Can you work these out from the model? Positions are in its coordinate system, mm. Coordinates: 2 decimals unless noted, no trailing zeros. Write each loop counter-clockwise with the first axis right and the second up, starting at its lowest first coordinate (ties: lowest second). Pieces come first, ordered by that corner, then holes. Notation, with made-up numbers: (-21.5, 79.25) -> (11.5, 79.25) arc R20 cw to (11.5, 88.25) -> close; hole circle Ø11 at (-33, -30). An arc over 180 degrees is marked (long way). Use one line per item in the form item = value.
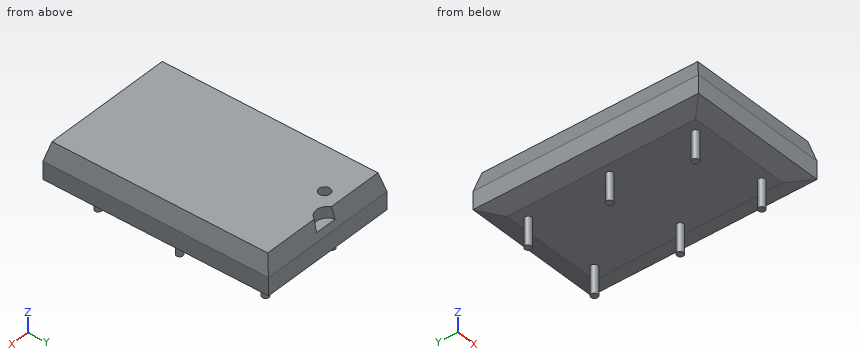
```python
from build123d import *
from OCP.BRepFilletAPI import BRepFilletAPI_MakeChamfer

# Parameters (mm, degrees)
SKETCH_2_W          = 12.6
SKETCH_2_H          = 20.2
EXTRUDE_1_DEPTH     = 3.68
CHAMFER_1_SIZE      = 1.65
CHAMFER_1_SIZE2     = 0.442116168
SKETCH_6_R          = 1
SKETCH_6_R_2        = 0.5
CUT_EXTRUDE_1_DEPTH = 1
SKETCH_7_R          = 0.3
EXTRUDE_2_DEPTH     = 2.5


with BuildPart() as part:
    # Эскиз2 → Вытянуть1 (new body)
    with BuildSketch(Plane.XY.offset(4.32)):
        with Locations((4.13, -7.62)):
            Rectangle(SKETCH_2_W, SKETCH_2_H)
    extrude(amount=-EXTRUDE_1_DEPTH)

    # Фаска1: one chamfer whose edges measure the first distance from different faces: ONE call of the kernel's chamfer builder (chamfer() names one face for all edges)
    chamfer_1_edges_1 = [part.edges().sort_by_distance(p)[0] for p in [
        (10.43, -7.62, 0.64),
        (4.13, 2.48, 0.64),
        (-2.17, -7.62, 0.64),
        (4.13, -17.72, 0.64),
    ]]
    chamfer_1_side_1 = [part.faces().sort_by_distance(p)[0] for p in [
        (4.13, -7.62, 0.64),
    ]]
    chamfer_1_edges_2 = [part.edges().sort_by_distance(p)[0] for p in [
        (4.13, 2.48, 4.32),
    ]]
    chamfer_1_side_2 = [part.faces().sort_by_distance(p)[0] for p in [
        (4.13, 2.48, 2.48),
    ]]
    chamfer_1_edges_3 = [part.edges().sort_by_distance(p)[0] for p in [
        (10.43, -7.62, 4.32),
    ]]
    chamfer_1_side_3 = [part.faces().sort_by_distance(p)[0] for p in [
        (10.43, -7.62, 2.48),
    ]]
    chamfer_1_edges_4 = [part.edges().sort_by_distance(p)[0] for p in [
        (4.13, -17.72, 4.32),
    ]]
    chamfer_1_side_4 = [part.faces().sort_by_distance(p)[0] for p in [
        (4.13, -17.72, 2.48),
    ]]
    chamfer_1_edges_5 = [part.edges().sort_by_distance(p)[0] for p in [
        (-2.17, -7.62, 4.32),
    ]]
    chamfer_1_side_5 = [part.faces().sort_by_distance(p)[0] for p in [
        (-2.17, -7.62, 2.48),
    ]]
    chamfer_1 = BRepFilletAPI_MakeChamfer(part.part.solid().wrapped)
    for e in chamfer_1_edges_1:
        chamfer_1.Add(CHAMFER_1_SIZE, CHAMFER_1_SIZE2, e.wrapped, chamfer_1_side_1[0].wrapped)  # the first distance lies on this face
    for e in chamfer_1_edges_2:
        chamfer_1.Add(CHAMFER_1_SIZE, CHAMFER_1_SIZE2, e.wrapped, chamfer_1_side_2[0].wrapped)  # the first distance lies on this face
    for e in chamfer_1_edges_3:
        chamfer_1.Add(CHAMFER_1_SIZE, CHAMFER_1_SIZE2, e.wrapped, chamfer_1_side_3[0].wrapped)  # the first distance lies on this face
    for e in chamfer_1_edges_4:
        chamfer_1.Add(CHAMFER_1_SIZE, CHAMFER_1_SIZE2, e.wrapped, chamfer_1_side_4[0].wrapped)  # the first distance lies on this face
    for e in chamfer_1_edges_5:
        chamfer_1.Add(CHAMFER_1_SIZE, CHAMFER_1_SIZE2, e.wrapped, chamfer_1_side_5[0].wrapped)  # the first distance lies on this face
    add(Compound.cast(chamfer_1.Shape()), mode=Mode.REPLACE)

    # Эскиз6 → Вырез-Вытянуть1 (cut)
    with BuildSketch(Plane.XY.offset(4.32)):
        with Locations((4.13, 2.48)):
            Circle(SKETCH_6_R)
        with Locations((2.197434959, 0.574075773)):
            Circle(SKETCH_6_R_2)
    extrude(amount=-CUT_EXTRUDE_1_DEPTH, mode=Mode.SUBTRACT)

    # Эскиз7 → Вытянуть2 (add)
    with BuildSketch(Plane(origin=(0, 0, 0.64), x_dir=(-1, 0, 0), z_dir=(0, 0, -1))):
        with Locations(Location((-7.88, -7.62, 0), (0, 0, 180))):
            Circle(SKETCH_7_R)
        with Locations(Location((-7.653482529, -0.12, 0), (0, 0, 180))):
            Circle(SKETCH_7_R)
        with Locations(Location((-7.653482529, -15.12, 0), (0, 0, 180))):
            Circle(SKETCH_7_R)
        with Locations(Location((-0.606517471, -15.12, 0), (0, 0, 180))):
            Circle(SKETCH_7_R)
        with Locations(Location((-0.606517471, -0.12, 0), (0, 0, 180))):
            Circle(SKETCH_7_R)
        with Locations(Location((-0.38, -7.62, 0), (0, 0, 180))):
            Circle(SKETCH_7_R)
    extrude(amount=EXTRUDE_2_DEPTH)


solid = part.part
```
Q1. Suppose I cut it at D-D (x = -1). Write out the boundary of the cut face in (y, z).
Return value:
outline = (-17.72, 1.08) -> (-16.55, 0.77) -> (1.31, 0.77) -> (2.48, 1.08) -> (2.48, 2.67) -> (2.04, 4.32) -> (-17.28, 4.32) -> (-17.72, 2.67) -> close
Q2. Suppose I cut it at B-B (y = -15.12). Write out the boundary of the cut face in (x, z).
Return value:
outline = (-2.17, 1.08) -> (-0.52, 0.64) -> (0.31, 0.64) -> (0.31, -1.86) -> (0.91, -1.86) -> (0.91, 0.64) -> (7.35, 0.64) -> (7.35, -1.86) -> (7.95, -1.86) -> (7.95, 0.64) -> (8.78, 0.64) -> (10.43, 1.08) -> (10.43, 2.67) -> (9.99, 4.32) -> (-1.73, 4.32) -> (-2.17, 2.67) -> close
Q3. Suppose I cut it at A-A (z = 0.25). Write out the boundary of the cut face in (x, y), then the cut area to 3 significant figures.
Return value:
outline = circle Ø0.6 at (0.38, -7.62); circle Ø0.6 at (0.61, -15.12); circle Ø0.6 at (0.61, -0.12); circle Ø0.6 at (7.65, -15.12); circle Ø0.6 at (7.65, -0.12); circle Ø0.6 at (7.88, -7.62)
area = 1.70 mm2
Q4. If I drill on line 1 (Z direction, x = 7, y = -6); line 2 (Z direction, x = 1, y = -16.5); line 3 (X direction, y = -13, z = 4), over which ranges is the centre line in solid material (lowest first)? Write a range as from..to.
Return value:
line_1 = 0.64..4.32
line_2 = 0.76..4.32
line_3 = -1.81..10.07
Q5. Suppose I cut it at C-C (z = 3.75). Write out the boundary of the cut face in (x, y).
Return value:
outline = (-1.88, -17.43) -> (10.14, -17.43) -> (10.14, 2.19) -> (5.09, 2.19) arc R1 cw to (3.17, 2.19) -> (-1.88, 2.19) -> close; hole circle Ø1 at (2.2, 0.57)
